from build123d import *

# Parameters (mm, degrees)
SKETCH1_W           = 33
SKETCH1_H           = 24
BOSS_EXTRUDE1_DEPTH = 3
SKETCH2_W           = 23
SKETCH2_H           = 12
SKETCH2_W_2         = 1.5
SKETCH2_H_2         = 5
SKETCH2_R           = 1.5
SKETCH2_W_3         = 12
SKETCH2_H_3         = 3
CUT_EXTRUDE1_DEPTH  = 4
SKETCH3_W           = 0.15
SKETCH3_H           = 3
SKETCH3_W_2         = 1.5
SKETCH3_H_2         = 5
CUT_EXTRUDE2_DEPTH  = 4


with BuildPart() as part:
    # Sketch1 → Boss-Extrude1 (new body)
    with BuildSketch(Plane(origin=(0, 0, 0), x_dir=(1, 0, 0), z_dir=(0, 1, 0))):
        with Locations((16.5, 12)):
            Rectangle(SKETCH1_W, SKETCH1_H)
    extrude(amount=BOSS_EXTRUDE1_DEPTH)

    # Sketch2 → Cut-Extrude1 (cut, through all)
    with BuildSketch(Plane(origin=(0, 3, 0), x_dir=(1, 0, 0), z_dir=(0, 1, 0))):
        with Locations((16.5, 12)):
            Rectangle(SKETCH2_W, SKETCH2_H)
        with Locations((28.75, 12)):
            Rectangle(SKETCH2_W_2, SKETCH2_H_2)
        with Locations((30, 21)):
            Circle(SKETCH2_R)
        with Locations((16.5, 4.5)):
            Rectangle(SKETCH2_W_3, SKETCH2_H_3)
        with Locations((16.5, 19.5)):
            Rectangle(SKETCH2_W_3, SKETCH2_H_3)
        with Locations((30, 3)):
            Circle(SKETCH2_R)
        with Locations((3, 3)):
            Circle(SKETCH2_R)
        with Locations((3, 21)):
            Circle(SKETCH2_R)
    extrude(amount=-CUT_EXTRUDE1_DEPTH, mode=Mode.SUBTRACT)

    # Sketch3 → Cut-Extrude2 (cut, through all)
    with BuildSketch(Plane(origin=(0, 3, 0), x_dir=(1, 0, 0), z_dir=(0, 1, 0))):
        with Locations((10.425, 19.5)):
            Rectangle(SKETCH3_W, SKETCH3_H)
        with Locations((22.575, 19.5)):
            Rectangle(SKETCH3_W, SKETCH3_H)
        with Locations((22.575, 4.5)):
            Rectangle(SKETCH3_W, SKETCH3_H)
        with Locations((10.425, 4.5)):
            Rectangle(SKETCH3_W, SKETCH3_H)
        with Locations((30.25, 12)):
            Rectangle(SKETCH3_W_2, SKETCH3_H_2)
    extrude(amount=-CUT_EXTRUDE2_DEPTH, mode=Mode.SUBTRACT)


solid = part.part
The model under review builds one solid part; all positions refer to its coordinate system, in mm. A direction names the side the tool comes from. Round coordinates to 2 decimals unless told otherwise and drop trailing zeros. Loops run counter-clockwise (first coordinate to the right, second up) from the corner with the lowest first, then second, coordinate; pieces in that order, holes last. Notation, with made-up numbers: M 61.25,5 L 85.25,5 A31 cw 85.25,43 Z; hole C -24.5,61 d10. An arc over 180 degrees is marked long. Answer as a JSON object with one key per item and string values.
Item 1: We need section D-D, the plane x = 30. State the section outline as (y, z) points.
Check sheet entries:
{"outline": "M 0,-24 L 3,-24 L 3,-22.5 L 0,-22.5 Z; M 0,-19.5 L 3,-19.5 L 3,-14.5 L 0,-14.5 Z; M 0,-9.5 L 3,-9.5 L 3,-4.5 L 0,-4.5 Z; M 0,-1.5 L 3,-1.5 L 3,0 L 0,0 Z"}
Item 2: Clearance check with a flat-ended pin moving along its axis: P1, Ø1.8, axis at x = 3, z = -3, coming from the +Y side. State where the tip first meets the part, or that it passes through.
Check sheet entries:
{"P1": "through"}
Item 3: We need section C-C, the plane y = 1.7. State the section outline as (x, z) points.
Check sheet entries:
{"outline": "M 0,-24 L 33,-24 L 33,0 L 0,0 Z; hole C 3,-21 d3; hole C 3,-3 d3; hole M 5,-18 L 10.35,-18 L 10.35,-21 L 22.65,-21 L 22.65,-18 L 28,-18 L 28,-14.5 L 31,-14.5 L 31,-9.5 L 28,-9.5 L 28,-6 L 22.65,-6 L 22.65,-3 L 10.35,-3 L 10.35,-6 L 5,-6 Z; hole C 30,-21 d3; hole C 30,-3 d3"}
Item 4: Tool access review of faces 1 (the face through (9, 3, -20)), 2 (the face through (29, 2, -9.5)): name each direction out of +Z, -Z, +X, -X, +Y, -Y from which nothing blocks a thin tool from reaching the whole face with its end or side.
Check sheet entries:
{"face 1": "+Z, -Z, +X, -X, +Y", "face 2": "+Y, -Y"}
Item 5: We need section A-A, the plane z = -7.75. State the section outline as (x, y) points, and give its area (3 significant figures).
Check sheet entries:
{"outline": "M 0,0 L 5,0 L 5,3 L 0,3 Z; M 28,0 L 33,0 L 33,3 L 28,3 Z", "area": "30.0 mm2"}
Item 6: We need section B-B, the plane x = 20. State the section outline as (y, z) points, and give its area (3 significant figures).
Check sheet entries:
{"outline": "M 0,-24 L 3,-24 L 3,-21 L 0,-21 Z; M 0,-3 L 3,-3 L 3,0 L 0,0 Z", "area": "18.0 mm2"}
Item 7: For line 1 along Z through (x, y) = (30, 2); line 2 along Z through (x, y) = (3, 1.05); line 3 along Z through (x, y) = (21, 0.9), list the stretches that pass through material, from the lowest coordinate up.
Check sheet entries:
{"line 1": "-24 to -22.5, -19.5 to -14.5, -9.5 to -4.5, -1.5 to 0", "line 2": "-24 to -22.5, -19.5 to -4.5, -1.5 to 0", "line 3": "-24 to -21, -3 to 0"}
